Check sheet for the drawn part. Datum: minimum x, y, z corner. Units: mm. Give positions to 0.01 mm unless a question says otherwise; leave off trailing zeros. Loops run counter-clockwise (first coordinate to the right, second up) from the corner with the lowest first, then second, coordinate; pieces in that order, holes last. Notation, with made-up numbers: (31.25, -10.5) - (65.25, -10.5) arc R16 cw to (65.25, -6.5) - close; hole circle Ø1 at (33, 71.25). An arc over 180 degrees is marked (long way). One line per item, written item: value. Start each with the question number.
1. Sectioned sample at B-B (y = 17.75). Record the cut outline in (x, z), plus the area to 3 significant figures.
2. Sectioned sample at C-C (x = 110). Record the cut outline in (y, z), plus the area to 3 significant figures.
3. Scan lines: L1, parallel to X at y = 18.5, z = 0.5; L2, parallel to Y at x = 111, z = 2.75. Record each from-to range of solid material in increasing order. Write a range as [from, to].
4. Sectioned sample at A-A (z = 0.55). Record the cut outline in (x, y).
5. Gauge pin test, flat ends, axial feed: pin 1 (0.9 mm diameter, centred on y = 2, z = 1.5, fed in from -X); pin 2 (0.9 mm diameter, centred on x = 2, z = 2, fed in from +Y); pin 3 (0.9 mm diameter, centred on y = 1.5, z = 1, fed in from +X). Record the tip position at first contact, or that the pin passes through.
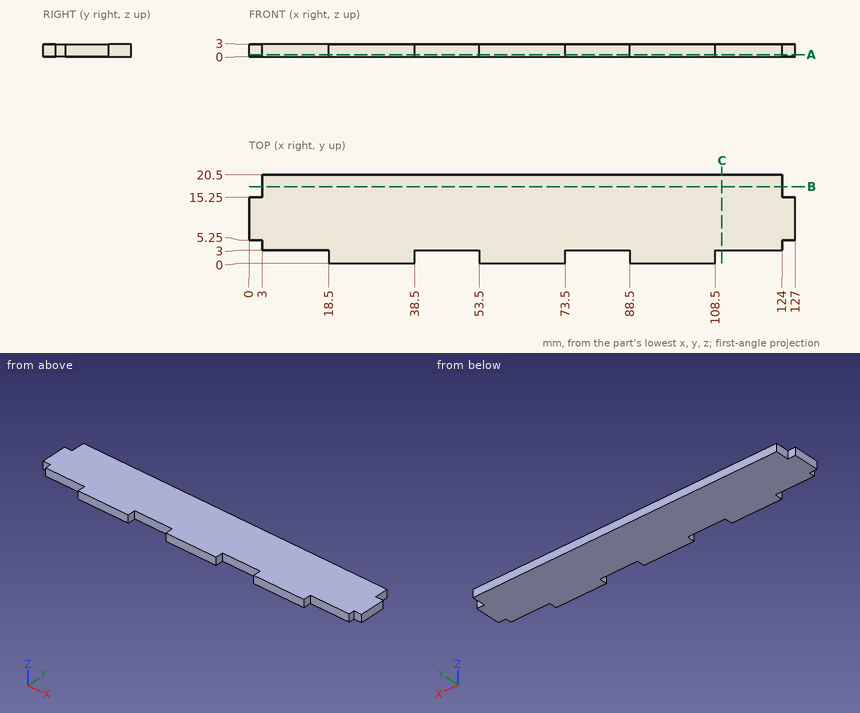
Results are:
1. outline: (3, 0) - (124, 0) - (124, 3) - (3, 3) - close
1. area: 363 mm^2
2. outline: (3, 0) - (20.5, 0) - (20.5, 3) - (3, 3) - close
2. area: 52.5 mm^2
3. L1: x = [3, 124]
3. L2: y = [3, 20.5]
4. outline: (0, 5.25) - (3, 5.25) - (3, 3) - (18.5, 3) - (18.5, 0) - (38.5, 0) - (38.5, 3) - (53.5, 3) - (53.5, 0) - (73.5, 0) - (73.5, 3) - (88.5, 3) - (88.5, 0) - (108.5, 0) - (108.5, 3) - (124, 3) - (124, 5.25) - (127, 5.25) - (127, 15.25) - (124, 15.25) - (124, 20.5) - (3, 20.5) - (3, 15.25) - (0, 15.25) - close
5. pin 1: stops at x = 18.5
5. pin 2: stops at y = 15.25
5. pin 3: stops at x = 108.5
